Can you work these out from the drawing? Everything is in mm from the part's minimum corner. Round coordinates to 2 decimals unless told otherwise and drop trailing zeros. Loops run counter-clockwise (first coordinate to the right, second up) from the corner with the lowest first, then second, coordinate; pieces in that order, holes last. Notation, with made-up numbers: M 75,-31 L 122,-31 A5 cw 122,-27 Z; hole C 13.5,15 d3. An arc over 180 degrees is marked long. One line per question, with ' | ' between items. Start each with the question number.
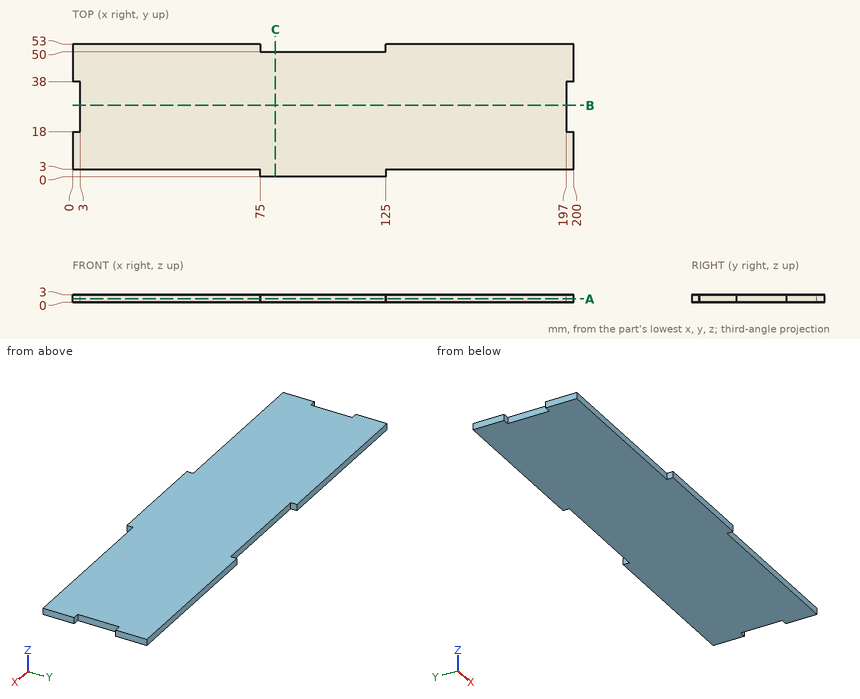
1) I'm going to push flat-ended pins straight in: pin 1 Ø0.9 at (y, z) = (1, 1) entering from -X; pin 2 Ø0.9 at (y, z) = (27.5, 1.5) entering from -X; pin 3 Ø0.9 at (y, z) = (1, 1) entering from +X. Where does each tip first touch, or does it pass through?
2) Please list where these lines run through material, in increasing order: L1, parallel to Y at x = 46, z = 2; L2, parallel to Y at x = 109, z = 2.15; L3, parallel to X at y = 31, z = 1.75. Write a range as from..to.
3) Imagine slicing it at B-B (y = 28.5). Write out the boundary of the cut face in (x, z), then the cut area to 3 significant figures.
4) Imagine slicing it at C-C (x = 81). Write out the boundary of the cut face in (y, z).
5) Imagine slicing it at A-A (z = 1.35). Write out the boundary of the cut face in (x, y), then the cut area to 3 significant figures.
Results are:
1) pin 1: x = 75 | pin 2: x = 3 | pin 3: x = 125
2) L1: 3..53 | L2: 0..50 | L3: 3..197
3) outline: M 3,0 L 197,0 L 197,3 L 3,3 Z | area: 582 mm²
4) outline: M 0,0 L 50,0 L 50,3 L 0,3 Z
5) outline: M 0,3 L 75,3 L 75,0 L 125,0 L 125,3 L 200,3 L 200,18 L 197,18 L 197,38 L 200,38 L 200,53 L 125,53 L 125,50 L 75,50 L 75,53 L 0,53 L 0,38 L 3,38 L 3,18 L 0,18 Z | area: 9,880 mm²
